Autodesk Inventor part; units mm, degrees
ref_plane "YZ Plane" through (0, 0, 0) normal (1, 0, 0) x (0, 1, 0)
ref_plane "XZ Plane" through (0, 0, 0) normal (0, 1, 0) x (-1, 0, 0)
ref_plane "XY Plane" through (0, 0, 0) normal (0, 0, 1) x (1, 0, 0)
sketch "Sketch2" plane through (0, 0, 0) normal (0, 1, 0) x (-1, 0, 0)
  line L0 (0, 0) -> (0, -149.1716)
  line L1 (-105.4802, 105.4802) -> (0, 0)
  line L2 (2, 0.8284) -> (2, -149.1716)
  line L3 (-104.066, 106.8944) -> (2, 0.8284)
  line L4 (-104.066, 106.8944) -> (-105.4802, 105.4802)
  line L5 (0, -149.1716) -> (2, -149.1716)
  line L6 (0, -200.3848) -> (0, 158.1076)
  dimension "d2" = 0
  dimension "d5" = 2
  dimension "d6" = 2
  dimension "d7" = 135
  dimension "d8" = 135
  dimension "d9" = 150
  dimension "d10" = 150
  dimension "d42" = 149.1716
  dimension "d43" = 149.1716
extrude "Extrusion1" add sketch "Sketch2" along normal blind 200
sketch "Sketch3" plane through (0, 0, 0) normal (0.7071, 0, -0.7071) x (-0.7071, 0, -0.7071)
  circle A0 centre (-136.6716, 50) radius 2.5
  line L0 (-149.1716, 0) -> (-149.1716, 200)
  line L1 (-149.1716, 0) -> (0, 0)
  circle A1 centre (-136.6716, 100) radius 2.5
  circle A2 centre (-136.6716, 150) radius 2.5
  line L2 (-149.1716, 200) -> (0, 200)
  dimension "d11" = 12.5
  dimension "d13" = 5
  dimension "d14" = 5
  dimension "d16" = 5
  dimension "d17" = 12.5
  dimension "d19" = 12.5
  dimension "d20" = 50
  dimension "d21" = 50
  dimension "d24" = 50
  dimension "d25" = 50
extrude "Extrusion2" cut sketch "Sketch3" against normal blind 3
sketch "Sketch4" plane through (0, 0, 0) normal (1, 0, 0) x (0, 0, -1)
  line L0 (149.1716, 0) -> (149.1716, 200)
  line L1 (0, 200) -> (149.1716, 200)
  line L2 (0, 0) -> (149.1716, 0)
  point P0 (136.6716, 150)
  point P1 (136.6716, 100)
  point P2 (136.6716, 50)
  dimension "d28" = 12.5
  dimension "d29" = 12.5
  dimension "d30" = 12.5
  dimension "d31" = 50
  dimension "d32" = 50
  dimension "d33" = 50
  dimension "d34" = 50
hole "Hole1" at (0, 150, -136.6716) at (0, 100, -136.6716) at (0, 50, -136.6716) direction (-1, 0, 0) diameter 5 end through all
properties part number "Thesis_part"
Input: part model. Units: mm. Frame: model coordinates. A direction names the side the tool comes from. Round coordinates to 2 decimals unless told otherwise and drop trailing zeros. Loops run counter-clockwise (first coordinate to the right, second up) from the corner with the lowest first, then second, coordinate; pieces in that order, holes last. Notation, with made-up numbers: (-21.5, 53.25) -> (-3.5, 53.25) arc R17 ccw to (-3.5, 65.25) -> close; hole circle Ø5 at (-33, -9). An arc over 180 degrees is marked (long way). Answer as a JSON object with one key per item and string values. Group by question number.
1) Reachability of faces 1 (the flat face through (0, 99, -74)), 2 (the flat face through (51.775, 98.6, 54.604)) from +Z, -Z, +X, -X, +Y, -Y: full face, straight path, thin tool, end or side. Return the list, or none.
2) Ray query, L1, parallel to X at y = 83, z = -109; L2, parallel to Z at x = -1, y = 100; L3, parallel to Z at x = -0.65, y = 150. Return the intervals inside material, ascending.
3) Section query B-B on z = 9.5. Output: boundary loops of the cut face in (x, y), plus the area to 3 significant figures.
4) Section query A-A on y = 30. Output: boundary loops of the cut face in (x, z), plus the area to 3 significant figures.
5) Pin query (flat end, axial travel): pin 1 (12 mm diameter, centred on y = 50, z = -20, fed in from +X); pin 2 (4 mm diameter, centred on x = 72.5, y = 100, fed in from +Z); pin 3 (4 mm diameter, centred on y = 91.5, z = 79.5, fed in from -X). Return the tip coordinate at first contact, or that it passes through.
6) Section query C-C on x = 5. Output: boundary loops of the cut face in (y, z).
Reply:
{
 "1": {"face 1": "-Z, +X, +Y, -Y", "face 2": "+Z, -X, +Y, -Y"},
 "2": {"L1": "x = -2 to 0", "L2": "z = -149.17 to -139.17, -134.17 to 1.83", "L3": "z = -149.17 to -139.17, -134.17 to 2.18"},
 "3": {"outline": "(6.67, 0) -> (9.5, 0) -> (9.5, 200) -> (6.67, 200) -> close", "area": "566 mm2"},
 "4": {"outline": "(-2, -149.17) -> (0, -149.17) -> (0, 0) -> (105.48, 105.48) -> (104.07, 106.89) -> (-2, 0.83) -> close", "area": "598 mm2"},
 "5": {"pin 1": "stops at x = 0", "pin 2": "stops at z = 77.33", "pin 3": "stops at x = 74.67"},
 "6": {"outline": "(0, 5) -> (200, 5) -> (200, 7.83) -> (0, 7.83) -> close"}
}
